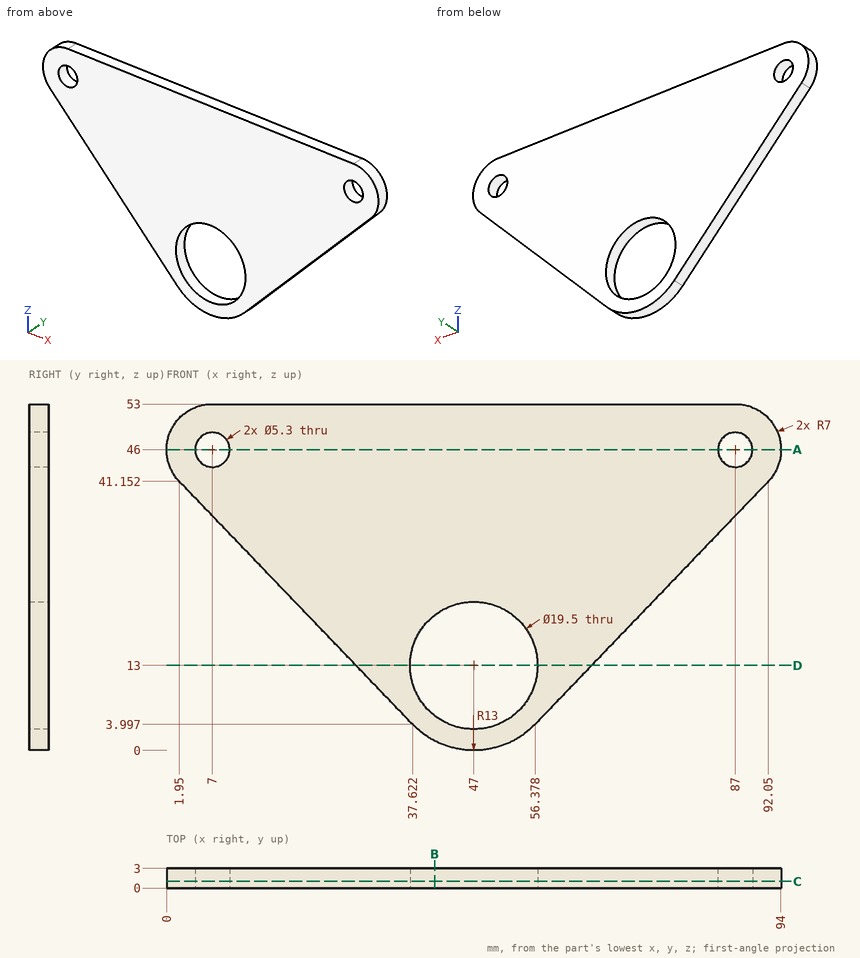
Geometry check sheet. Reference: drawing and pictorial views, mm from the part's lowest x, y, z. Round coordinates to 2 decimals unless told otherwise and drop trailing zeros. Write each loop counter-clockwise with the first axis right and the second up, starting at its lowest first coordinate (ties: lowest second). Pieces come first, ordered by that corner, then holes.
Item 1: Section check B-B (x = 41). Record the boundary of the cut face in (y, z) (1 decimal).
Determined:
outline: (0, 1.5) - (3, 1.5) - (3, 5.3) - (0, 5.3) - close; (0, 20.7) - (3, 20.7) - (3, 53) - (0, 53) - close
Item 2: Go/stop test with a flat-tipped pin: pin 1 Ø1 at (x, y) = (40, 0.5) entering from -Z. Record where the tip stops, or that it passes through.
Determined:
pin 1: stops at z = 1.74
Item 3: Material ranges on line 1 along X through (y, z) = (1.05, 46); line 2 along X through (y, z) = (1.3, 48); line 3 along Z through (x, y) = (47.5, 2.45), recorded low to high.
Determined:
line 1: x = 0 to 4.35, 9.65 to 84.35, 89.65 to 94
line 2: x = 0.29 to 5.26, 8.74 to 85.26, 88.74 to 93.71
line 3: z = 0.01 to 3.26, 22.74 to 53
Item 4: Section check C-C (y = 1). Record the boundary of the cut face in (x, z).
Determined:
outline: (1.95, 41.15) - (37.62, 4) arc R13 ccw to (56.38, 4) - (92.05, 41.15) arc R7 ccw to (87, 53) - (7, 53) arc R7 ccw to start; hole circle Ø5.3 at (7, 46); hole circle Ø19.5 at (47, 13); hole circle Ø5.3 at (87, 46)
Item 5: Section check D-D (z = 13). Record the boundary of the cut face in (x, y).
Determined:
outline: (28.98, 0) - (37.25, 0) - (37.25, 3) - (28.98, 3) - close; (56.75, 0) - (65.02, 0) - (65.02, 3) - (56.75, 3) - close
Item 6: Section check A-A (z = 46). Record the boundary of the cut face in (x, y).
Determined:
outline: (0, 0) - (4.35, 0) - (4.35, 3) - (0, 3) - close; (9.65, 0) - (84.35, 0) - (84.35, 3) - (9.65, 3) - close; (89.65, 0) - (94, 0) - (94, 3) - (89.65, 3) - close
